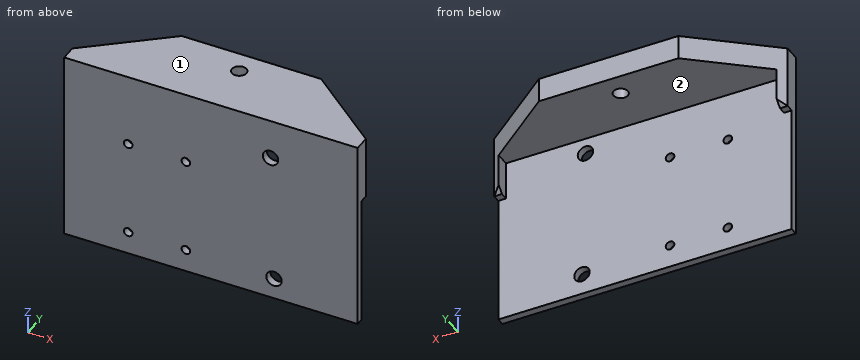
```python
from build123d import *

# Parameters (mm, degrees)
BOSS_EXTRUDE1_DEPTH      = 2.54
BOSS_EXTRUDE1_DEPTH_BACK = 2.54
SKETCH1_W                = 69.85
SKETCH1_H                = 63.5
SKETCH1_R                = 1.4224
SKETCH1_R_2              = 2.54
SKETCH2_W                = 69.85
SKETCH2_H                = 8.038671265
BOSS_EXTRUDE2_DEPTH      = 20.32
BOSS_EXTRUDE3_DEPTH      = 2.54
BOSS_EXTRUDE4_DEPTH      = 2.54
SKETCH5_W                = 42.761328735
SKETCH5_H                = 2.54
CUT_EXTRUDE1_DEPTH       = 89.142435188
SKETCH6_W                = 69.85
SKETCH6_H                = 2.54
BOSS_EXTRUDE5_DEPTH      = 12.7
SKETCH7_W                = 69.85
SKETCH7_H                = 2.54
CUT_EXTRUDE2_DEPTH       = 12.7
SKETCH8_R                = 2.38125
CUT_EXTRUDE3_DEPTH       = 96.449847624
BOSS_EXTRUDE6_DEPTH      = 10.922
BOSS_EXTRUDE7_DEPTH      = 10.922
CUT_EXTRUDE4_DEPTH       = 10.922
CUT_EXTRUDE5_DEPTH       = 10.922
CUT_EXTRUDE6_DEPTH       = 104.461914585
CUT_EXTRUDE6_DEPTH_BACK  = 104.461914585


with BuildPart() as part:
    # Sketch1 → Boss-Extrude1 (new, two sides: drawn at the far end of the back side and taken through both)
    with BuildSketch(Plane(origin=(0, 0, 0), x_dir=(1, 0, 0), z_dir=(0, 1, 0)).offset(-BOSS_EXTRUDE1_DEPTH_BACK)):
        with Locations((30.031991128, 8.648073975)):
            Rectangle(SKETCH1_W, SKETCH1_H)
        with Locations(Location((2.726991128, 32.778073975, 0), (0, 0, 270))):
            Circle(SKETCH1_R, mode=Mode.SUBTRACT)
        with Locations(Location((21.776991128, 32.778073975, 0), (0, 0, 270))):
            Circle(SKETCH1_R, mode=Mode.SUBTRACT)
        with Locations(Location((2.726991128, 1.028073975, 0), (0, 0, 270))):
            Circle(SKETCH1_R, mode=Mode.SUBTRACT)
        with Locations(Location((21.776991128, 1.028073975, 0), (0, 0, 270))):
            Circle(SKETCH1_R, mode=Mode.SUBTRACT)
        with Locations(Location((49.680840227, -9.802293314, 0), (0, 0, 270))):
            Circle(SKETCH1_R_2, mode=Mode.SUBTRACT)
        with Locations(Location((50.825492869, 33.377706686, 0), (0, 0, 270))):
            Circle(SKETCH1_R_2, mode=Mode.SUBTRACT)
    extrude(amount=BOSS_EXTRUDE1_DEPTH + BOSS_EXTRUDE1_DEPTH_BACK)

    # Sketch2 → Boss-Extrude2 (add)
    with BuildSketch(Plane(origin=(0, 2.54, 0), x_dir=(1, 0, 0), z_dir=(0, 1, 0))):
        with Locations((30.031991128, -19.082590393)):
            Rectangle(SKETCH2_W, SKETCH2_H)
    extrude(amount=BOSS_EXTRUDE2_DEPTH)

    # Sketch3 → Boss-Extrude3 (add)
    with BuildSketch(Plane.ZY.offset(4.893008872)):
        Polygon((15.06325476, 15.24), (2.36325476, 2.54), (-40.398073975, 2.54), (-40.398073975, -2.54), (23.101926025, -2.54), (23.101926025, 22.86), (15.06325476, 22.86), align=None)
    extrude(amount=BOSS_EXTRUDE3_DEPTH)

    # Sketch4 → Boss-Extrude4 (add)
    with BuildSketch(Plane(origin=(64.956991128, 0, 0), x_dir=(0, 0, -1), z_dir=(1, 0, 0))):
        Polygon((-15.06325476, 15.24), (-2.36325476, 2.54), (40.398073975, 2.54), (40.398073975, -2.54), (-23.101926025, -2.54), (-23.101926025, 22.86), (-15.06325476, 22.86), align=None)
    extrude(amount=BOSS_EXTRUDE4_DEPTH)

    # Sketch5 → Cut-Extrude1 (cut, through all)
    with BuildSketch(Plane.ZY.offset(7.433008872)):
        with Locations((-19.017409607, 1.27)):
            Rectangle(SKETCH5_W, SKETCH5_H)
    extrude(amount=-CUT_EXTRUDE1_DEPTH, mode=Mode.SUBTRACT)

    # Sketch6 → Boss-Extrude5 (add)
    with BuildSketch(Plane(origin=(0, 0, 2.36325476), x_dir=(-1, 0, 0), z_dir=(0, 0, -1))):
        with Locations((-30.031991128, 1.27)):
            Rectangle(SKETCH6_W, SKETCH6_H)
    extrude(amount=-BOSS_EXTRUDE5_DEPTH)

    # Sketch7 → Cut-Extrude2 (cut)
    with BuildSketch(Plane(origin=(0, 0, 2.36325476), x_dir=(-1, 0, 0), z_dir=(0, 0, -1))):
        with Locations((-30.031991128, 1.27)):
            Rectangle(SKETCH7_W, SKETCH7_H)
    extrude(amount=-CUT_EXTRUDE2_DEPTH, mode=Mode.SUBTRACT)

    # Sketch8 → Cut-Extrude3 (cut, through all)
    with BuildSketch(Plane.XY.offset(23.101926025)):
        with Locations((30.031991128, 15.24)):
            Circle(SKETCH8_R)
    extrude(amount=-CUT_EXTRUDE3_DEPTH, mode=Mode.SUBTRACT)

    # Sketch9 → Boss-Extrude6 (add)
    with BuildSketch(Plane(origin=(67.496991128, 0, 0), x_dir=(0, 0, -1), z_dir=(1, 0, 0))):
        Polygon((-2.36325476, 0), (-2.36325476, 2.54), (-15.06325476, 15.24), (-15.06325476, 22.86), (-23.101926025, 22.86), (-23.101926025, -2.54), (40.398073975, -2.54), (40.398073975, 0), align=None)
    extrude(amount=BOSS_EXTRUDE6_DEPTH)

    # Sketch10 → Boss-Extrude7 (add)
    with BuildSketch(Plane.ZY.offset(7.433008872)):
        Polygon((2.36325476, 2.54), (2.36325476, 0), (-40.398073975, 0), (-40.398073975, -2.54), (23.101926025, -2.54), (23.101926025, 22.86), (15.06325476, 22.86), (15.06325476, 15.24), align=None)
    extrude(amount=BOSS_EXTRUDE7_DEPTH)

    # Sketch12 → Cut-Extrude4 (cut)
    with BuildSketch(Plane.ZY.offset(-64.956991128)):
        Polygon((15.06325476, 15.24), (2.36325476, 2.54), (2.36325476, 0), (15.06325476, 0), align=None)
    extrude(amount=-CUT_EXTRUDE4_DEPTH, mode=Mode.SUBTRACT)

    # Sketch13 → Cut-Extrude5 (cut)
    with BuildSketch(Plane(origin=(-4.893008872, 0, 0), x_dir=(0, 0, -1), z_dir=(1, 0, 0))):
        Polygon((-2.36325476, 2.54), (-15.06325476, 15.24), (-15.06325476, 0), (-2.36325476, 0), align=None)
    extrude(amount=-CUT_EXTRUDE5_DEPTH, mode=Mode.SUBTRACT)

    # Sketch14 → Cut-Extrude6 (cut, two sides: drawn at the far end of the back side and taken through both)
    with BuildSketch(Plane.XY.offset(23.101926025).offset(-CUT_EXTRUDE6_DEPTH_BACK)):
        Polygon((78.418991128, 22.86), (53.018991128, 22.86), (78.418991128, 2.54), align=None)
        Polygon((-18.355008872, 22.86), (7.044991128, 22.86), (-18.355008872, 2.54), align=None)
    extrude(amount=CUT_EXTRUDE6_DEPTH + CUT_EXTRUDE6_DEPTH_BACK, mode=Mode.SUBTRACT)


solid = part.part
```
Part model, mm, in its own coordinate system. Face numbers are marked on the shaded views. A direction names the side the tool comes from. Round coordinates to 2 decimals unless told otherwise and drop trailing zeros. Order: outer loops, then holes, each group sorted by start corner. A loop starts at its lowest first (then second) coordinate and runs counter-clockwise, first axis right, second up. Notation, with made-up numbers: M 5,16 L 54,16 A11 ccw 54,26 Z; hole C 81,-30.75 d10. An arc over 180 degrees is marked long. Answer in a Markdown table with one row per item. Add a question column.
Q1. Cut at C-C on y = 1.5. Give the cut face in (x, z) (3 decimals).
Q2. 3-axis set-ups, long thin cutter, end or side, ignore diameter. For the marked faces 1 and 2: which of +Z, -Z, +X, -X, +Y, -Y reach the whole face in a straight line?
Q3. Pin check, flat tips, straight feed: pin 1 (2 mm diameter, centred on x = 20, z = -13.5, fed in from +Y); pin 2 (12 mm diameter, centred on y = 8, z = -18, fed in from +X); pin 3 (2 mm diameter, centred on x = -17.5, y = 2, fed in from -Z). Stop position of each tip, or through.
Q4. Cut at D-D on z = -17. Give the cut face in (x, y) (3 decimals), and give its area (3 significant figures).
Q5. Cut at B-B on z = -1. Give the cut face in (x, y) (3 decimals).
Q6. Cut at A-A on y = 15.24. Give the cut face in (x, z).
Q7. Wall check: L1, parallel to Z at x = 56.5, y = 16.5; L2, parallel to Y at x = 72, z = -18; L3, parallel to Y at x = 30, z = 20.5. Give the ranges that are in metal, low to high. Write a range as from..to.
Established:
| question | item | result |
|---|---|---|
| 1 | outline | M -18.355,2.363 L -15.815,2.363 L -15.815,15.063 L 75.879,15.063 L 75.879,2.363 L 78.419,2.363 L 78.419,23.102 L -18.355,23.102 Z |
| 2 | face 1 | +Z, +X, -X, +Y, -Y |
| 2 | face 2 | -Z, +Y |
| 3 | pin 1 | stops at y = 0 |
| 3 | pin 2 | passes through |
| 3 | pin 3 | stops at z = 2.36 |
| 4 | outline | M -18.355,-2.54 L 78.419,-2.54 L 78.419,0 L -18.355,0 Z |
| 4 | area | 246 mm2 |
| 5 | outline | M -18.355,-2.54 L 1.305,-2.54 L 1.305,0 L -18.355,0 Z; M 4.149,-2.54 L 20.355,-2.54 L 20.355,0 L 4.149,0 Z; M 23.199,-2.54 L 78.419,-2.54 L 78.419,0 L 23.199,0 Z |
| 6 | outline | M -2.48,15.06 L 27.65,15.06 L 27.65,23.1 L -2.48,23.1 Z; M 32.41,15.06 L 62.54,15.06 L 62.54,23.1 L 32.41,23.1 Z |
| 7 | L1 | z = 15.06..23.1 |
| 7 | L2 | y = -2.54..0 |
| 7 | L3 | y = -2.54..12.86, 17.62..22.86 |
